from build123d import *

# Parameters (mm, degrees)
SKETCH2_R                = 2
BOSS_EXTRUDE1_DEPTH      = 1.5
BOSS_EXTRUDE1_DEPTH_BACK = 1.5
SKETCH3_R                = 1
CUT_EXTRUDE1_DEPTH       = 50


with BuildPart() as part:
    # Sketch1 → Revolve1 (revolve)
    with BuildSketch(Plane.XY):
        Polygon((0, 0), (-9, 0), (-9, 9), (-8.5, 10), (-8.5, 58), (-9, 58), (-9, 78), (-7.5, 78), (-7.5, 2), (0, 2), align=None)
    revolve(axis=Axis((0, 78, 0), (0, -1, 0)))

    # Sketch2 → Boss-Extrude1 (add, two sides)
    with BuildSketch(Plane.XY) as boss_extrude1_sk:
        with BuildLine():
            Line((-7, 0), (7, 0))
            Line((7, 0), (7, -6))
            ThreePointArc((7, -6), (0, -13), (-7, -6))
            Line((-7, -6), (-7, 0))
        make_face()
        with Locations((0, -6)):
            Circle(SKETCH2_R, mode=Mode.SUBTRACT)
    extrude(amount=BOSS_EXTRUDE1_DEPTH)
    extrude(boss_extrude1_sk.sketch, amount=-BOSS_EXTRUDE1_DEPTH_BACK)

    # Sketch3 → Cut-Extrude1 (cut)
    with BuildSketch(Plane(origin=(0, 0, 0), x_dir=(0, 0, -1), z_dir=(1, 0, 0))):
        with Locations((0, 65)):
            Circle(SKETCH3_R)
        with Locations((0, 4)):
            Circle(SKETCH3_R)
    extrude(amount=CUT_EXTRUDE1_DEPTH, mode=Mode.SUBTRACT)


solid = part.part
Can you work these out from the model? Positions are in its coordinate system, mm. A direction names the side the tool comes from. Give positions to 0.01 mm unless a question says otherwise; leave off trailing zeros. Loops run counter-clockwise (first coordinate to the right, second up) from the corner with the lowest first, then second, coordinate; pieces in that order, holes last. Notation, with made-up numbers: (31, 87) -> (83, 87) arc R25 cw to (83, 101) -> close; hole circle Ø10 at (45, 26). An arc over 180 degrees is marked (long way). Write item = value, one per line.
1) For faces 1 (the flat face through (0, 2, 0)), 2 (the flat face through (-1, -8, 1.5)), 3 (the flat face through (8, 58, 3.3)), which set-ups out of +Z, -Z, +X, -X, +Y, -Y let a thin tool reach every point of the face, with its end or its side?
Check result:
face_1 = +Y
face_2 = +Z, +X, -X, -Y
face_3 = none
2) Thinking about a two-plate mould opening in Z: for faces 4 (the flat face through (-1, -8, -1.5)), 5 (the cylindrical face through (8, 64, 0)), 6 (the cylindrical face through (0, -13, 0)), which applies, released by +Z, released by -Z, zero draft, split by the parting line, or undercut?
Check result:
face_4 = released by -Z
face_5 = undercut
face_6 = zero draft
3) Suppose I cut it at A-A on y = 61.5. Write out the boundary of the cut face in (x, z).
Check result:
outline = circle Ø18 at (0, 0); hole circle Ø15 at (0, 0)
4) I need wall thicknesses on L1, parallel to Z at x = 0.25, y = 73; L2, parallel to X at y = 47, z = -0.5; L3, parallel to Y at x = -3.25, z = 7.75. Which ranges of each line are inside material? Lowest first, please. Write a range as from..to.
Check result:
L1 = -9..-7.5, 7.5..9
L2 = -8.49..-7.48, 7.48..8.49
L3 = 0..78
5) Suppose I cut it at B-B on y = 30. Write out the boundary of the cut face in (x, z).
Check result:
outline = circle Ø17 at (0, 0); hole circle Ø15 at (0, 0)
6) Will these pins go through, and if not, where does the flat tip stop? pin 1 (5 mm diameter, centred on x = 1, y = 9.5, fed in from -Z); pin 2 (1 mm diameter, centred on y = 4.5, z = -3.5, fed in from -X); pin 3 (1 mm diameter, centred on x = -6, z = -1.5, fed in from -Y); pin 4 (5 mm diameter, centred on x = 0, y = -6, fed in from -Z).
Check result:
pin_1 = -9
pin_2 = -8.49
pin_3 = -10.33
pin_4 = -1.5
